Autodesk Inventor part; units mm, degrees
ref_plane "YZ Plane" through (0, 0, 0) normal (1, 0, 0) x (0, 1, 0)
ref_plane "XZ Plane" through (0, 0, 0) normal (0, 1, 0) x (-1, 0, 0)
ref_plane "XY Plane" through (0, 0, 0) normal (0, 0, 1) x (1, 0, 0)
sketch "Sketch1" plane through (0, 0, 0) normal (0, 0, 1) x (1, 0, 0)
  line L0 (-25, 12.5) -> (25, 12.5)
  line L1 (25, 12.5) -> (25, -12.5)
  line L2 (25, -12.5) -> (-25, -12.5)
  line L3 (-25, -12.5) -> (-25, 12.5)
  point P0 (0, 0)
  point P1 (0, 12.5)
  point P2 (-25, 0)
  dimension "d0" = 50
  dimension "d1" = 25
extrude "Extrusion1" add sketch "Sketch1" along normal blind 18
sketch "Sketch5" plane through (0, 0, 18) normal (0, 0, 1) x (1, 0, 0)
  line L0 (2.5, 8.5) -> (-12.5, 8.5) construction
  line L1 (2.5, 10.25) -> (-12.5, 10.25)
  line L2 (-12.5, 6.75) -> (2.5, 6.75)
  arc A0 (2.5, 6.75) -> (2.5, 10.25) centre (2.5, 8.5) ccw
  arc A1 (-12.5, 10.25) -> (-12.5, 6.75) centre (-12.5, 8.5) ccw
  line L3 (2.5, -8.5) -> (-12.5, -8.5) construction
  line L4 (2.5, -6.75) -> (-12.5, -6.75)
  line L5 (-12.5, -10.25) -> (2.5, -10.25)
  arc A2 (2.5, -10.25) -> (2.5, -6.75) centre (2.5, -8.5) ccw
  arc A3 (-12.5, -6.75) -> (-12.5, -10.25) centre (-12.5, -8.5) ccw
  line L6 (25, 12.5) -> (-25, 12.5)
  line L7 (-25, -12.5) -> (25, -12.5)
  line L8 (-25, 12.5) -> (-25, -12.5)
  point P0 (0, 0)
  point P1 (-5, 8.5)
  point P2 (-5, -8.5)
  dimension "d29" = 3.5
  dimension "d30" = 4
  dimension "d31" = 4
  dimension "d32" = 20
  dimension "d33" = 15
extrude "Extrusion5" cut sketch "Sketch5" against normal through all contours A2 L5 A3 L4
sketch "Sketch6" plane through (0, 0, 18) normal (0, 0, 1) x (1, 0, 0)
  line L0 (15, 0) -> (-25, 0)
  line L1 (-25, 0) -> (-25, 12.5)
  line L2 (-25, 12.5) -> (15, 12.5)
  line L3 (15, 12.5) -> (15, 0)
  line L4 (25, -12.5) -> (25, 12.5)
  line L5 (-25, 12.5) -> (-25, -12.5)
  line L6 (25, 12.5) -> (-25, 12.5)
  point P0 (0, 0)
  dimension "d36" = 10
extrude "Extrusion6" cut sketch "Sketch6" against normal through all
sketch "Sketch7" plane through (0, 0, 18) normal (0, 0, 1) x (1, 0, 0)
  line L0 (15, -12.5) -> (-25, -12.5)
  line L1 (-25, -12.5) -> (-25, 0)
  line L2 (-25, 0) -> (15, 0)
  line L3 (15, 0) -> (15, -12.5)
  line L4 (15, 12.5) -> (15, 0)
  line L5 (-25, -12.5) -> (25, -12.5)
  line L6 (-25, 0) -> (-25, -12.5)
  line L7 (15, 0) -> (-25, 0)
  point P0 (0, 0)
  point P1 (15, 2)
  point P2 (13, 0)
extrude "Extrusion7" cut sketch "Sketch7" against normal blind 10
fillet "Fillet2" radius 2 1 edges at (15, 0, 4)
properties part number "0005-10-025 Activator senzor Y"
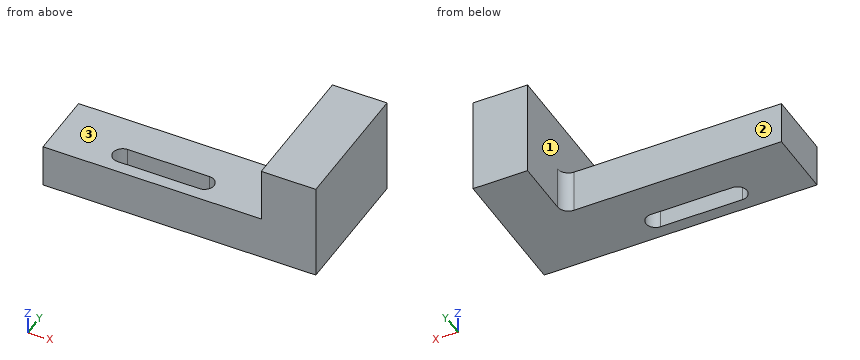
The listing builds one solid part. Answer for the finished solid, in the listing's coordinates (mm). Face numbers are marked on the shaded views. A direction names the side the tool comes from. Round coordinates to 2 decimals unless told otherwise and drop trailing zeros. Order: outer loops, then holes, each group sorted by start corner. A loop starts at its lowest first (then second) coordinate and runs counter-clockwise, first axis right, second up. Notation, with made-up numbers: (21, 9) -> (36, 9) arc R9 ccw to (36, 26) -> close; hole circle Ø8 at (52, -26.75). An arc over 180 degrees is marked (long way). Write each question's results on one line, items separated by ' | '. Start each with the question number.
Q1. Find section B-B (x = -10). Determine the outline of the cut face in (y, z).
Q2. Find section D-D (z = 11.75). Determine the outline of the cut face in (x, y).
Q3. Straight lines are drawn through the part: probe 1 along Y at (x, z) = (2, 3.5); probe 2 along X at (y, z) = (7.5, 12.75); probe 3 along Z at (x, y) = (-4, -1.75). For each, find the intervals that lie inside material, in ascending order. Write a range as from..to.
Q4. Find section A-A (y = -8.5). Determine the outline of the cut face in (x, z).
Q5. Find section C-C (x = -19). Determine the outline of the cut face in (y, z).
Q6. Which of the six approach directions +Z, -Z, +X, -X, +Y, -Y give full straight-line access (tool end or side, diameter ignored) to the marked faces 1, 2 and 3?
Q7. Each of these flat-tipped pins is pushed along its axis until it touches: pin 1 (4 mm diameter, centred on x = -8, y = -5, fed in from +Z); pin 2 (2.5 mm diameter, centred on x = -7, z = 4, fed in from +Y). Where does it stop, or does it pass through?
Worked answers:
1) outline: (-12.5, 0) -> (-10.25, 0) -> (-10.25, 8) -> (-12.5, 8) -> close; (-6.75, 0) -> (0, 0) -> (0, 8) -> (-6.75, 8) -> close
2) outline: (15, -12.5) -> (25, -12.5) -> (25, 12.5) -> (15, 12.5) -> close
3) probe 1: y = -12.5..-10.25, -6.75..0 | probe 2: x = 15..25 | probe 3: z = 0..8
4) outline: (-25, 0) -> (-14.25, 0) -> (-14.25, 8) -> (-25, 8) -> close; (4.25, 0) -> (25, 0) -> (25, 18) -> (15, 18) -> (15, 8) -> (4.25, 8) -> close
5) outline: (-12.5, 0) -> (0, 0) -> (0, 8) -> (-12.5, 8) -> close
6) face 1: +Z, -X, +Y | face 2: +Z, -Z, -X, +Y | face 3: +Z, -X, +Y, -Y
7) pin 1: stops at z = 8 | pin 2: stops at y = 0
